Could you check a few things on this drawing? It's one solid part, dimensions in mm from its lowest x, y, z. Give positions to 0.01 mm unless a question says otherwise; leave off trailing zeros. Write each loop counter-clockwise with the first axis right and the second up, starting at its lowest first coordinate (ties: lowest second). Pieces come first, ordered by that corner, then holes. Notation, with made-up numbers: M 59,-10.75 L 92,-10.75 A24 ccw 92,24.25 Z; hole C -16.5,59 d8. An arc over 180 degrees is marked long. Answer as CSV lines item,"result". Start each with the question number.
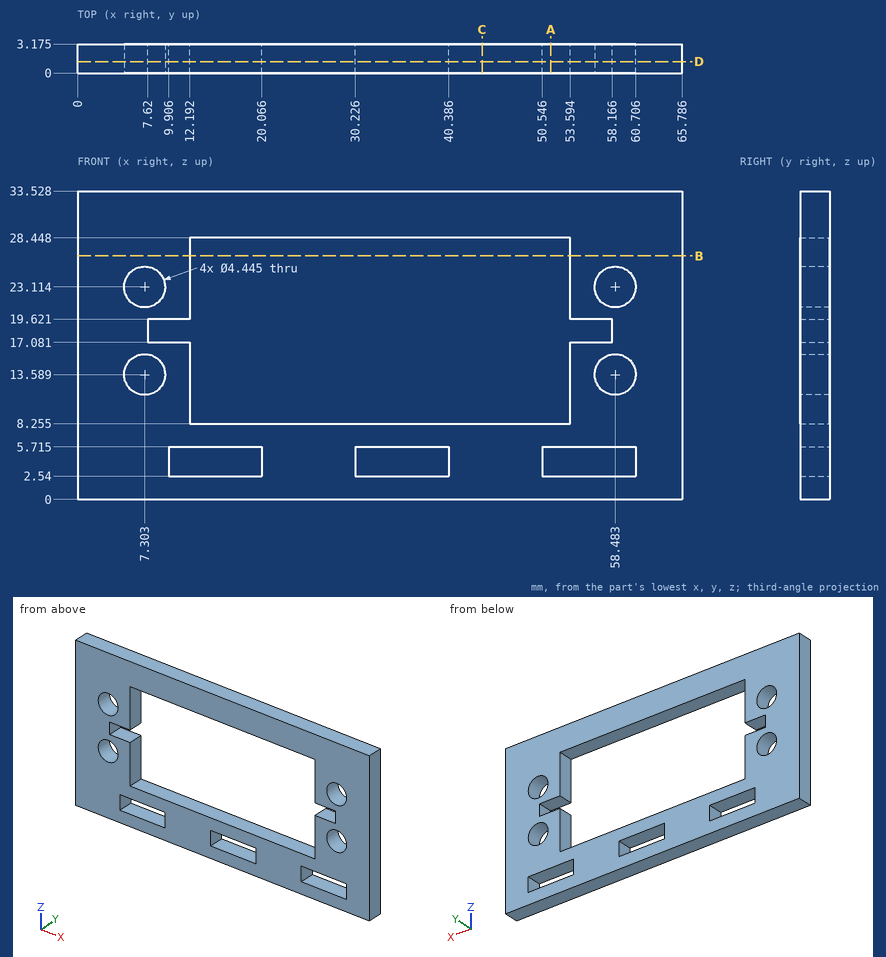
1) I want a section at C-C, the plane x = 44. Please give me the cut outline in (y, z) (1 decimal).
2) I want a section at B-B, the plane z = 26.5. Please give me the cut outline in (x, y) (1 decimal).
3) I want a section at A-A, the plane x = 51.5. Please give me the cut outline in (y, z) (1 decimal).
4) I'm going to push flat-ended pins straight in: P1, Ø7, axis at x = 58.48, z = 23.11, coming from the -Y side; P2, Ø1.5, axis at x = 34, z = 10.5, coming from the +Y side. Where does each tip first touch, or does it pass through?
5) I want a section at D-D, the plane y = 1.25. State how many separate pieces and enclosed holes the cut face has, then the cut area to 3 significant figures.
6) I need wall thicknesses on L1, parallel to Z at x = 11.5, y = 1.55 (1 decimal); L2, parallel to Z at x = 36.5, y = 1.65 (1 decimal); L3, parallel to X at y = 0.2, z = 18 (1 decimal). Which ranges of each line are inside material? Lowest first, please. Write a range as from..to.
Values found:
1,outline,"M 0,0 L 3.2,0 L 3.2,8.3 L 0,8.3 Z; M 0,28.4 L 3.2,28.4 L 3.2,33.5 L 0,33.5 Z"
2,outline,"M 0,0 L 12.2,0 L 12.2,3.2 L 0,3.2 Z; M 53.6,0 L 65.8,0 L 65.8,3.2 L 53.6,3.2 Z"
3,outline,"M 0,0 L 3.2,0 L 3.2,2.5 L 0,2.5 Z; M 0,5.7 L 3.2,5.7 L 3.2,8.3 L 0,8.3 Z; M 0,28.4 L 3.2,28.4 L 3.2,33.5 L 0,33.5 Z"
4,P1,"stops at y = 0"
4,P2,"passes through"
5,separate pieces,"1"
5,enclosed holes,"8"
5,area,"1,190 mm²"
6,L1,"z = 0..2.5, 5.7..17.1, 19.6..33.5"
6,L2,"z = 0..2.5, 5.7..8.3, 28.4..33.5"
6,L3,"x = 0..7.6, 58.2..65.8"
